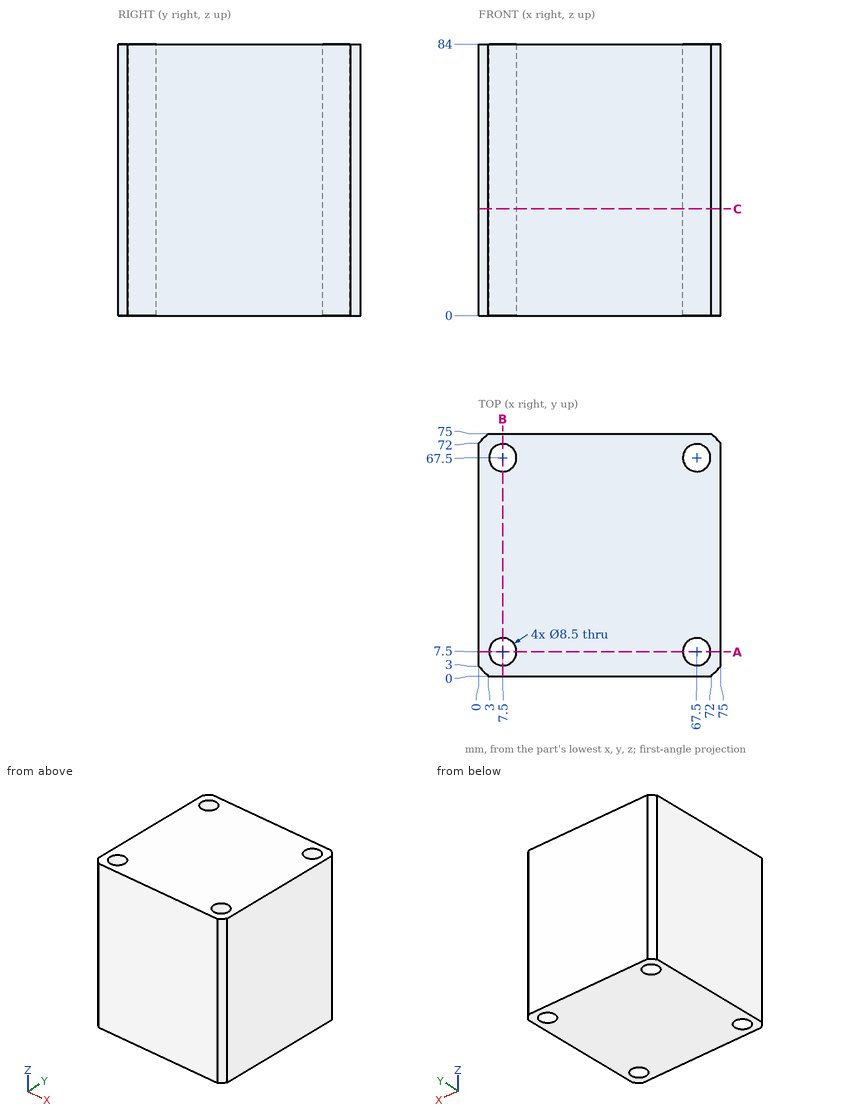
Geometry: see drawing. Coordinates: mm, zero at the bounding-box minimum. Give positions to 0.01 mm unless a question says otherwise; leave off trailing zeros. Order: outer loops, then holes, each group sorted by start corner. A loop starts at its lowest first (then second) coordinate and runs counter-clockwise, first axis right, second up. Notation, with made-up numbers: M -15,-9 L 4,-9 A12 ccw 4,-4 Z; hole C 47.25,37.5 d7. An arc over 180 degrees is marked long. Answer as a JSON object with one key per item and string values.
1. Ray query, line 1 (Y direction, x = 7.5, z = 61); line 2 (Y direction, x = 66, z = 53.5); line 3 (X direction, y = 7, z = 21). Return the intervals inside material, ascending. Write a range as [from, to].
Result sheet:
{"line 1": "[0, 3.25], [11.75, 63.25], [71.75, 75]", "line 2": "[0, 3.52], [11.48, 63.52], [71.48, 75]", "line 3": "[0, 3.28], [11.72, 63.28], [71.72, 75]"}
2. Cut plane A-A, the plane y = 7.5. Output: boundary loops of the cut face in (x, z), and give its area (3 significant figures).
Result sheet:
{"outline": "M 0,0 L 3.25,0 L 3.25,84 L 0,84 Z; M 11.75,0 L 63.25,0 L 63.25,84 L 11.75,84 Z; M 71.75,0 L 75,0 L 75,84 L 71.75,84 Z", "area": "4,870 mm²"}
3. First-contact query: P1, Ø5, axis at x = 7.5, y = 67.5, coming from the -Z side. Flat tip, straight axial feed; report the tip coordinate or a pass-through.
Result sheet:
{"P1": "through"}
4. Cut plane C-C, the plane z = 33. Output: boundary loops of the cut face in (x, y), and give its area (3 significant figures).
Result sheet:
{"outline": "M 0,3 L 3,0 L 72,0 L 75,3 L 75,72 L 72,75 L 3,75 L 0,72 Z; hole C 7.5,7.5 d8.5; hole C 7.5,67.5 d8.5; hole C 67.5,7.5 d8.5; hole C 67.5,67.5 d8.5", "area": "5,380 mm²"}
